Autodesk Inventor part; units mm, degrees
ref_plane "YZ Plane" through (0, 0, 0) normal (1, 0, 0) x (0, 1, 0)
ref_plane "XZ Plane" through (0, 0, 0) normal (0, 1, 0) x (-1, 0, 0)
ref_plane "XY Plane" through (0, 0, 0) normal (0, 0, 1) x (1, 0, 0)
sketch "PanelBody" plane through (0, 0, 0) normal (0, 0, 1) x (1, 0, 0)
  line L0 (-106.0995, -38.4223) -> (33.9005, -38.4223)
  line L1 (33.9005, -38.4223) -> (33.9005, -132.4223)
  line L2 (33.9005, -132.4223) -> (-106.0995, -132.4223)
  line L3 (-106.0995, -132.4223) -> (-106.0995, -38.4223)
  dimension "d1" = 140
  dimension "d2" = 94
extrude "PanelFace" add sketch "PanelBody" along normal blind 2
sketch "SideHooks" plane through (-106.0995, -132.4223, 0) normal (-1, 0, 0) x (0, 0, 1)
  line L0 (0, 94) -> (-1.9, 94)
  line L1 (-1.9, 94) -> (-1.9, 92.1)
  line L2 (-1.9, 92.1) -> (0, 92.1)
  line L3 (0, 92.1) -> (0, 94)
  line L4 (0, 0) -> (-1.9, 0)
  line L5 (-1.9, 0) -> (-1.9, 1.9)
  line L6 (-1.9, 1.9) -> (0, 1.9)
  line L7 (0, 1.9) -> (0, 0)
  point P0 (0, 132.4223)
  dimension "d33" = 1.9
extrude "Corners" add sketch "SideHooks" against normal blind 140
sketch "Sketch3" plane through (33.9005, -38.4223, -1.9) normal (0, 0, -1) x (-1, 0, 0)
  line L0 (0, -94) -> (140, -94) construction
  line L1 (140, -94) -> (140, 0) construction
  line L2 (140, 0) -> (0, 0) construction
  line L3 (0, 0) -> (0, -94) construction
  line L4 (137.5, -91.5) -> (133.8633, -91.5) construction
  line L5 (72.5, -86.5) -> (72.5, -56.6362)
  line L6 (137.5, -54.5) -> (137.5, -85.1873)
  line L7 (137.5, -2.5) -> (133.8633, -2.5) construction
  line L8 (72.5, -7.5) -> (72.5, -37.3638)
  line L9 (137.5, -39.5) -> (137.5, -8.8127)
  line L10 (2.5, -2.5) -> (6.1367, -2.5) construction
  line L11 (67.5, -7.5) -> (67.5, -37.3638)
  line L12 (2.5, -39.5) -> (2.5, -8.8127)
  line L13 (2.5, -91.5) -> (6.1367, -91.5) construction
  line L14 (67.5, -86.5) -> (67.5, -56.6362)
  line L15 (2.5, -54.5) -> (2.5, -85.1873)
  line L16 (72.5, -2.5) -> (67.5, -2.5) construction
  line L17 (2.5, -44.5) -> (2.5, -49.5) construction
  line L18 (67.5, -91.5) -> (72.5, -91.5) construction
  line L19 (137.5, -44.5) -> (137.5, -49.5) construction
  line L20 (135.2172, -7.5332) -> (79.3341, -41.7204)
  line L21 (74.7828, -38.6434) -> (129.3198, -5.2796)
  line L22 (65.2172, -38.6434) -> (10.6802, -5.2796)
  line L23 (60.6659, -41.7204) -> (4.7828, -7.5332)
  line L24 (11.4629, -2.5) -> (62.5, -2.5)
  line L25 (2.5, -6.1367) -> (2.5, -2.5) construction
  line L26 (80.1169, -44.5) -> (132.5, -44.5)
  line L27 (137.5, -6.1367) -> (137.5, -2.5) construction
  line L28 (128.5371, -2.5) -> (77.5, -2.5)
  line L29 (59.8831, -44.5) -> (7.5, -44.5)
  line L30 (135.2172, -86.4668) -> (79.3341, -52.2796)
  line L31 (74.7828, -55.3566) -> (129.3198, -88.7204)
  line L32 (65.2172, -55.3566) -> (10.6802, -88.7204)
  line L33 (4.7828, -86.4668) -> (60.6659, -52.2796)
  line L34 (80.1169, -49.5) -> (132.5, -49.5)
  line L35 (59.8831, -49.5) -> (7.5, -49.5)
  line L36 (2.5, -87.8633) -> (2.5, -91.5) construction
  line L37 (11.4629, -91.5) -> (62.5, -91.5)
  line L38 (128.5371, -91.5) -> (77.5, -91.5)
  line L39 (137.5, -87.8633) -> (137.5, -91.5) construction
  line L40 (140, -94) -> (0, -94)
  line L41 (140, 0) -> (0, 0)
  line L42 (0, -1.9) -> (0, -92.1)
  line L43 (140, 0) -> (140, -1.9)
  line L44 (103.0028, -27.2408) -> (100.3935, -22.9756) construction
  line L45 (91.7427, -59.8707) -> (89.1334, -64.1358) construction
  line L46 (57.5593, -60.0415) -> (54.95, -55.7763) construction
  line L47 (48.3721, -34.1995) -> (50.9813, -29.9344) construction
  line L48 (74.7906, -49.5) -> (65.2094, -49.5) construction
  line L49 (65.2094, -44.5) -> (74.7906, -44.5) construction
  line L50 (72.5, -53.9601) -> (72.5, -40.0399) construction
  line L51 (67.5, -53.9601) -> (67.5, -40.0399) construction
  arc A0 (77.5, -2.5) -> (72.5, -7.5) centre (77.5, -7.5) ccw
  arc A1 (67.5, -7.5) -> (62.5, -2.5) centre (62.5, -7.5) ccw
  arc A2 (72.5, -86.5) -> (77.5, -91.5) centre (77.5, -86.5) ccw
  arc A3 (62.5, -91.5) -> (67.5, -86.5) centre (62.5, -86.5) ccw
  arc A4 (2.5, -39.5) -> (7.5, -44.5) centre (7.5, -39.5) ccw
  arc A5 (7.5, -49.5) -> (2.5, -54.5) centre (7.5, -54.5) ccw
  arc A6 (137.5, -54.5) -> (132.5, -49.5) centre (132.5, -54.5) ccw
  arc A7 (132.5, -44.5) -> (137.5, -39.5) centre (132.5, -39.5) ccw
  arc A8 (80.1169, -49.5) -> (79.3341, -52.2796) centre (80.1169, -51) ccw
  arc A9 (74.7828, -55.3566) -> (72.5, -56.6362) centre (74, -56.6362) ccw
  arc A10 (67.5, -56.6362) -> (65.2172, -55.3566) centre (66, -56.6362) ccw
  arc A11 (60.6659, -52.2796) -> (59.8831, -49.5) centre (59.8831, -51) ccw
  arc A12 (59.8831, -44.5) -> (60.6659, -41.7204) centre (59.8831, -43) ccw
  arc A13 (65.2172, -38.6434) -> (67.5, -37.3638) centre (66, -37.3638) ccw
  arc A14 (72.5, -37.3638) -> (74.7828, -38.6434) centre (74, -37.3638) ccw
  arc A15 (79.3341, -41.7204) -> (80.1169, -44.5) centre (80.1169, -43) ccw
  arc A16 (137.5, -8.8127) -> (135.2172, -7.5332) centre (136, -8.8127) ccw
  arc A17 (129.3198, -5.2796) -> (128.5371, -2.5) centre (128.5371, -4) ccw
  arc A18 (11.4629, -2.5) -> (10.6802, -5.2796) centre (11.4629, -4) ccw
  arc A19 (4.7828, -7.5332) -> (2.5, -8.8127) centre (4, -8.8127) ccw
  arc A20 (2.5, -85.1873) -> (4.7828, -86.4668) centre (4, -85.1873) ccw
  arc A21 (10.6802, -88.7204) -> (11.4629, -91.5) centre (11.4629, -90) ccw
  arc A22 (128.5371, -91.5) -> (129.3198, -88.7204) centre (128.5371, -90) ccw
  arc A23 (135.2172, -86.4668) -> (137.5, -85.1873) centre (136, -85.1873) ccw
  dimension "d16" = 2.5
  dimension "d24" = 5
  dimension "d25" = 5
  dimension "d26" = 2.5
  dimension "d27" = 2.5
  dimension "d28" = 2.5
  dimension "d34" = 0
  dimension "d36" = 0
  dimension "d37" = 0
  dimension "d38" = 0
  dimension "d39" = 5
  dimension "d40" = 5
  dimension "d41" = 1.5
extrude "ReinforcementBars" cut sketch "Sketch3" against normal blind 3.2
sketch "Sketch4" plane through (0, 0, 2) normal (0, 0, 1) x (1, 0, 0)
  line L0 (-62.4757, -113.2868) -> (-62.4757, -58.6034) construction
  line L1 (-62.4757, -58.6034) -> (1.9126, -58.6034) construction
  line L2 (1.9126, -58.6034) -> (1.9126, -113.2868) construction
  line L3 (1.9126, -113.2868) -> (-62.4757, -113.2868) construction
  point P0 (0, 0)
extrude "Extrusion4" [suppressed]
properties part number "SidePanelNarrow" material "Nylon 6"
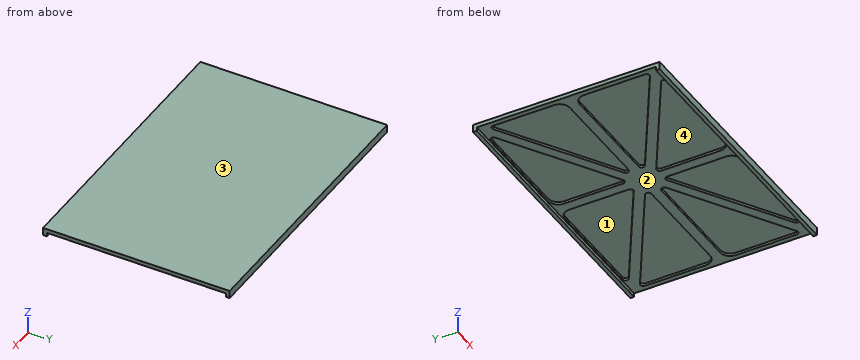
Verification items for the finished model (mm, model axes). Face numbers are marked on the shaded views. A direction names the side the tool comes from. Coordinates: 2 decimals unless noted, no trailing zeros. Order: outer loops, then holes, each group sorted by start corner. A loop starts at its lowest first (then second) coordinate and runs counter-clockwise, first axis right, second up. Notation, with made-up numbers: (-12, 67.25) -> (36, 67.25) arc R26 ccw to (36, 91.25) -> close; hole circle Ø10 at (12.25, -9). An arc over 180 degrees is marked (long way). Use CSV: the item, a comma, the result in double quotes. Start each with the question number.
Q1. Section check D-D, the plane x = -57.5. Record the cut outline in (y, z), and give its area (3 significant figures).
Q2. Tool access check on the marked faces 3 and 4. Record the directions out of +Z, -Z, +X, -X, +Y, -Y that give a thin tool (end or side, any length) a straight path to the whole face; none if there is none.
Q3. Section check A-A, the plane z = -0.85. Record the cut outline in (x, y).
Q4. Section check B-B, the plane y = -67. Record the cut outline in (x, z), and give its area (3 significant figures).
Q5. Draft check along X on the marked faces 1 and 2. Enter one of: +X half, -X half, draft (parallel to the pull), parting line (faces both ways), or undercut.
Q6. Depth check by flat-ended pin: P1, Ø18.5, axis at x = -11, y = -115, coming from the -Z side; P2, Ø8, axis at x = -27, y = -69.5, coming from the -Z side. Enter the tip coordinate at first touch or a pass-through.
Q7. Section check C-C, the plane x = -78. Record the cut outline in (y, z).
Q8. Thickness scan on line 1 along Y through (x, z) = (25.5, -0.4); line 2 along X through (y, z) = (-68.5, 0.4) (1 decimal); line 3 along Y through (x, z) = (-72.5, 0.3). Record the ranges inside material, lowest first.
Returned:
1,outline,"(-132.42, -1.9) -> (-130.52, -1.9) -> (-130.52, 0) -> (-129.92, 0) -> (-129.92, 1.3) -> (-103.95, 1.3) -> (-103.95, 0) -> (-98.08, 0) -> (-98.08, 1.3) -> (-87.92, 1.3) -> (-87.92, 0) -> (-82.92, 0) -> (-82.92, 1.3) -> (-72.76, 1.3) -> (-72.76, 0) -> (-66.9, 0) -> (-66.9, 1.3) -> (-40.92, 1.3) -> (-40.92, 0) -> (-40.32, 0) -> (-40.32, -1.9) -> (-38.42, -1.9) -> (-38.42, 2) -> (-132.42, 2) -> close"
1,area,"101 mm^2"
2,face 3,"+Z, +X, -X, +Y, -Y"
2,face 4,"-Z"
3,outline,"(-106.1, -132.42) -> (33.9, -132.42) -> (33.9, -130.52) -> (-106.1, -130.52) -> close; (-106.1, -40.32) -> (33.9, -40.32) -> (33.9, -38.42) -> (-106.1, -38.42) -> close"
4,outline,"(-106.1, 0) -> (-103.6, 0) -> (-103.6, 1.3) -> (-66.92, 1.3) -> (-66.92, 0) -> (-57.34, 0) -> (-57.34, 1.3) -> (-38.6, 1.3) -> (-38.6, 0) -> (-33.6, 0) -> (-33.6, 1.3) -> (-14.86, 1.3) -> (-14.86, 0) -> (-5.28, 0) -> (-5.28, 1.3) -> (31.4, 1.3) -> (31.4, 0) -> (33.9, 0) -> (33.9, 2) -> (-106.1, 2) -> close"
4,area,"136 mm^2"
5,face 1,"undercut"
5,face 2,"draft"
6,P1,"stops at z = 0"
6,P2,"stops at z = 1.3"
7,outline,"(-132.42, -1.9) -> (-130.52, -1.9) -> (-130.52, 0) -> (-129.92, 0) -> (-129.92, 1.3) -> (-116.49, 1.3) -> (-116.49, 0) -> (-110.62, 0) -> (-110.62, 1.3) -> (-87.92, 1.3) -> (-87.92, 0) -> (-82.92, 0) -> (-82.92, 1.3) -> (-60.22, 1.3) -> (-60.22, 0) -> (-54.36, 0) -> (-54.36, 1.3) -> (-40.92, 1.3) -> (-40.92, 0) -> (-40.32, 0) -> (-40.32, -1.9) -> (-38.42, -1.9) -> (-38.42, 2) -> (-132.42, 2) -> close"
8,line 1,"y = -132.42 to -130.52, -40.32 to -38.42"
8,line 2,"x = -106.1 to -103.6, -64.5 to -54.9, -38.6 to -33.6, -17.3 to -7.7, 31.4 to 33.9"
8,line 3,"y = -132.42 to -129.92, -113.12 to -107.26, -87.92 to -82.92, -63.58 to -57.72, -40.92 to -38.42"
